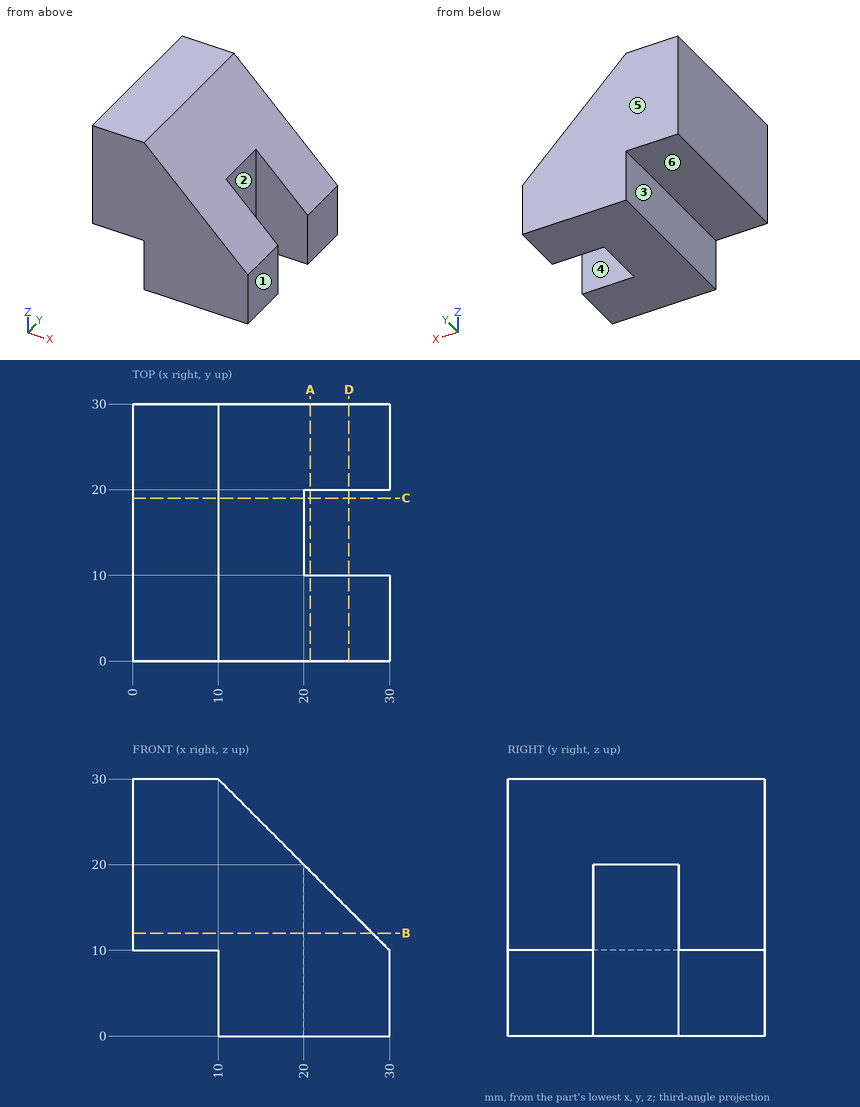
Source: three-view drawing plus pictorial views. Frame: mm from the lowest corner of the part. A direction names the side the tool comes from. Give positions to 0.01 mm unless a question says otherwise; leave off trailing zeros. Order: outer loops, then holes, each group sorted by start corner. A loop starts at its lowest first (then second) coordinate and runs counter-clockwise, first axis right, second up. Notation, with made-up numbers: (85.25, -0.75) -> (107.25, -0.75) arc R28 cw to (107.25, 38.25) -> close; hole circle Ø6 at (-39, -21.75). An arc over 180 degrees is marked (long way). Put each result on its own line as item: value.
Q1. Draft query along Y for the marked faces 4, 5 and 6. Return one class per face: released by +Y, released by -Y, zero draft, split by the parting line, or undercut.
Here are the results:
face 4: undercut
face 5: released by +Y
face 6: zero draft
Q2. Section C-C, the plane y = 19. Return loops of the section in (x, z).
Here are the results:
outline: (0, 10) -> (10, 10) -> (10, 0) -> (20, 0) -> (20, 20) -> (10, 30) -> (0, 30) -> close
Q3. Section B-B, the plane z = 12. Return loops of the section in (x, y), then the cut area to 3 significant figures.
Here are the results:
outline: (0, 0) -> (28, 0) -> (28, 10) -> (20, 10) -> (20, 20) -> (28, 20) -> (28, 30) -> (0, 30) -> close
area: 760 mm^2
Q4. Reachability of the marked faces 1, 2 and 3 from +Z, -Z, +X, -X, +Y, -Y: full face, straight path, thin tool, end or side. Return the list, or none.
Here are the results:
face 1: +Z, -Z, +X, +Y, -Y
face 2: +Z, -Z, +X
face 3: -Z, -X, +Y, -Y
Q5. Material intervals for L1, parallel to Y at x = 23, z = 9; L2, parallel to X at y = 18.5, z = 7.5; L3, parallel to X at y = 8.75, z = 9.5, sorted ascending.
Here are the results:
L1: y = 0 to 10, 20 to 30
L2: x = 10 to 20
L3: x = 10 to 30
Q6. Pin query (flat end, axial travel): pin 1 (5 mm diameter, centred on y = 16.5, z = 6, fed in from +X); pin 2 (4 mm diameter, centred on x = 19.5, z = 25.5, fed in from +Y); pin 3 (4 mm diameter, centred on x = 4.5, y = 15, fed in from -Z); pin 4 (10 mm diameter, centred on y = 25, z = 3.5, fed in from -X). Return the tip coordinate at first contact, or that it passes through.
Here are the results:
pin 1: stops at x = 20
pin 2: passes through
pin 3: stops at z = 10
pin 4: stops at x = 10
Q7. Section D-D, the plane x = 25.25. Return loops of the section in (y, z).
Here are the results:
outline: (0, 0) -> (10, 0) -> (10, 14.75) -> (0, 14.75) -> close; (20, 0) -> (30, 0) -> (30, 14.75) -> (20, 14.75) -> close
Q8. Section A-A, the plane x = 20.75. Return loops of the section in (y, z).
Here are the results:
outline: (0, 0) -> (10, 0) -> (10, 19.25) -> (0, 19.25) -> close; (20, 0) -> (30, 0) -> (30, 19.25) -> (20, 19.25) -> close
